from build123d import *

# Parameters (mm, degrees)
SKETCH1_W           = 45
SKETCH1_H           = 45
SKETCH1_R           = 2.25
BOSS_EXTRUDE1_DEPTH = 3
BOSS_EXTRUDE2_DEPTH = 20
CHAMFER1_SIZE       = 15
SKETCH4_R           = 2.25
CUT_EXTRUDE1_DEPTH  = 20
CUT_EXTRUDE2_DEPTH  = 3
SKETCH6_W           = 45
SKETCH6_H           = 10
CUT_EXTRUDE3_DEPTH  = 10


with BuildPart() as part:
    # Sketch1 → Boss-Extrude1 (new body)
    with BuildSketch(Plane.XY):
        Rectangle(SKETCH1_W, SKETCH1_H)
        with Locations((-15, 5)):
            Circle(SKETCH1_R, mode=Mode.SUBTRACT)
        with Locations((15, 5)):
            Circle(SKETCH1_R, mode=Mode.SUBTRACT)
        with Locations((15, -15)):
            Circle(SKETCH1_R, mode=Mode.SUBTRACT)
        with Locations((-15, -15)):
            Circle(SKETCH1_R, mode=Mode.SUBTRACT)
    extrude(amount=BOSS_EXTRUDE1_DEPTH)

    # Sketch3 → Boss-Extrude2 (add)
    with BuildSketch(Plane(origin=(0, -22.5, 0), x_dir=(-1, 0, 0), z_dir=(0, -1, 0))):
        with BuildLine():
            Line((7.5, -3), (-7.5, -3))
            Line((-7.5, -3), (-7.5, -50))
            ThreePointArc((-7.5, -50), (0, -57.5), (7.5, -50))
            Line((7.5, -50), (7.5, -3))
        make_face()
        with BuildLine():
            Line((1, -46.02382093), (1, -21.02382093))
            Line((1, -21.02382093), (-1, -21.02382093))
            Line((-1, -21.02382093), (-1, -46.02382093))
            ThreePointArc((-1, -46.02382093), (0, -54.1), (1, -46.02382093))
        make_face(mode=Mode.SUBTRACT)
    extrude(amount=-BOSS_EXTRUDE2_DEPTH)

    # Chamfer1
    chamfer1_edges = [part.edges().sort_by_distance(p)[0] for p in [
        (0, -2.5, 3),
    ]]
    chamfer(chamfer1_edges, length=CHAMFER1_SIZE)

    # Sketch4 → Cut-Extrude1 (cut)
    with BuildSketch(Plane.ZY.offset(7.5)):
        with Locations((34, -12.5)):
            Circle(SKETCH4_R)
    extrude(amount=-CUT_EXTRUDE1_DEPTH, mode=Mode.SUBTRACT)

    # Sketch5 → Cut-Extrude2 (cut)
    with BuildSketch(Plane(origin=(7.5, 0, 0), x_dir=(0, 0, -1), z_dir=(1, 0, 0))):
        Polygon((-34, -16.830127019), (-30.25, -14.665063509), (-30.25, -10.334936491), (-34, -8.169872981), (-37.75, -10.334936491), (-37.75, -14.665063509), align=None)
    extrude(amount=-CUT_EXTRUDE2_DEPTH, mode=Mode.SUBTRACT)

    # Sketch6 → Cut-Extrude3 (cut)
    with BuildSketch(Plane.XY.offset(3)):
        with Locations((0, 17.5)):
            Rectangle(SKETCH6_W, SKETCH6_H)
    extrude(amount=-CUT_EXTRUDE3_DEPTH, mode=Mode.SUBTRACT)


solid = part.part
Design review of the part built by this model. Coordinates are the model's own, in mm. A direction names the side the tool comes from. Give positions to 0.01 mm unless a question says otherwise; leave off trailing zeros. Write each loop counter-clockwise with the first axis right and the second up, starting at its lowest first coordinate (ties: lowest second). Pieces come first, ordered by that corner, then holes. Notation, with made-up numbers: M -27.75,-17 L -4.75,-17 A8 ccw -4.75,-9 Z; hole C 81,-30.75 d9. An arc over 180 degrees is marked long. Answer as a JSON object with one key per item and string values. Group by question number.
1) For line 1 along X through (y, z) = (-9.5, 43.5); line 2 along Z through (x, y) = (0, -13); line 3 along X through (y, z) = (-11, 50), list the stretches that pass through material, from the lowest coordinate up.
2) Clearance check with flat-ended pins moving along their axes: pin 1 Ø7.5 at (x, z) = (0, 50) entering from -Y; pin 2 Ø6 at (y, z) = (-10.5, 39.5) entering from +X; pin 3 Ø6 at (x, y) = (-15, 5) entering from +Z; pin 4 Ø17.5 at (y, z) = (-9.5, 25.5) entering from -X. State where each tip first meets the part, or that it passes through.
3) We need section C-C (z = 39.5). Give the boundary of the cut face in (x, y), and give its area (3 significant figures).
4) Mouldability with a two-part tool opening along Y and no side actions: class faces 5 (the face through (16.038, -16.996, 1.479)), 6 (the face through (-0.1, 4.9, 10.6)), 7 (the face through (7.5, -13, 26)) as released by +Y, released by -Y, zero draft, split by the parting line, or undercut.
5) Tool access review of faces 1 (the face through (-7.5, -13, 27)), 2 (the face through (0, -13, 21.024)), 3 (the face through (6.021, -15.732, 35.901)), 4 (the face through (2, -2.5, 37)): name each direction out of +Z, -Z, +X, -X, +Y, -Y from which nothing blocks a thin tool from reaching the whole face with its end or side.
6) We need section B-B (x = 15). Give the boundary of the cut face in (y, z).
7) We need section A-A (x = 0). Give the boundary of the cut face in (y, z), and give its area (3 significant figures).
8) We need section D-D (y = 5). Give the boundary of the cut face in (x, z).
Answer key:
{
 "1": {"line 1": "x = -7.5 to -1, 1 to 7.5", "line 2": "z = 0 to 21.02, 54.1 to 57.5", "line 3": "x = -7.5 to -4.1, 4.1 to 7.5"},
 "2": {"pin 1": "passes through", "pin 2": "stops at x = 7.5", "pin 3": "stops at z = 3", "pin 4": "stops at x = -7.5"},
 "3": {"outline": "M -7.5,-22.5 L -1,-22.5 L -1,-2.5 L -7.5,-2.5 Z; M 1,-22.5 L 7.5,-22.5 L 7.5,-2.5 L 1,-2.5 Z", "area": "260 mm²"},
 "4": {"face 5": "undercut", "face 6": "released by +Y", "face 7": "zero draft"},
 "5": {"face 1": "+Z, -X, +Y, -Y", "face 2": "+Y, -Y", "face 3": "+X", "face 4": "+Z, +X, -X, +Y"},
 "6": {"outline": "M -22.5,0 L -17.25,0 L -17.25,3 L -22.5,3 Z; M -12.75,0 L 2.75,0 L 2.75,3 L -12.75,3 Z; M 7.25,0 L 12.5,0 L 12.5,3 L 7.25,3 Z"},
 "7": {"outline": "M -22.5,0 L 12.5,0 L 12.5,3 L -2.5,18 L -2.5,21.02 L -22.5,21.02 Z; M -22.5,54.1 L -2.5,54.1 L -2.5,57.5 L -22.5,57.5 Z", "area": "646 mm²"},
 "8": {"outline": "M -22.5,0 L -17.25,0 L -17.25,3 L -22.5,3 Z; M -12.75,0 L 12.75,0 L 12.75,3 L 7.5,3 L 7.5,10.5 L -7.5,10.5 L -7.5,3 L -12.75,3 Z; M 17.25,0 L 22.5,0 L 22.5,3 L 17.25,3 Z"}
}
